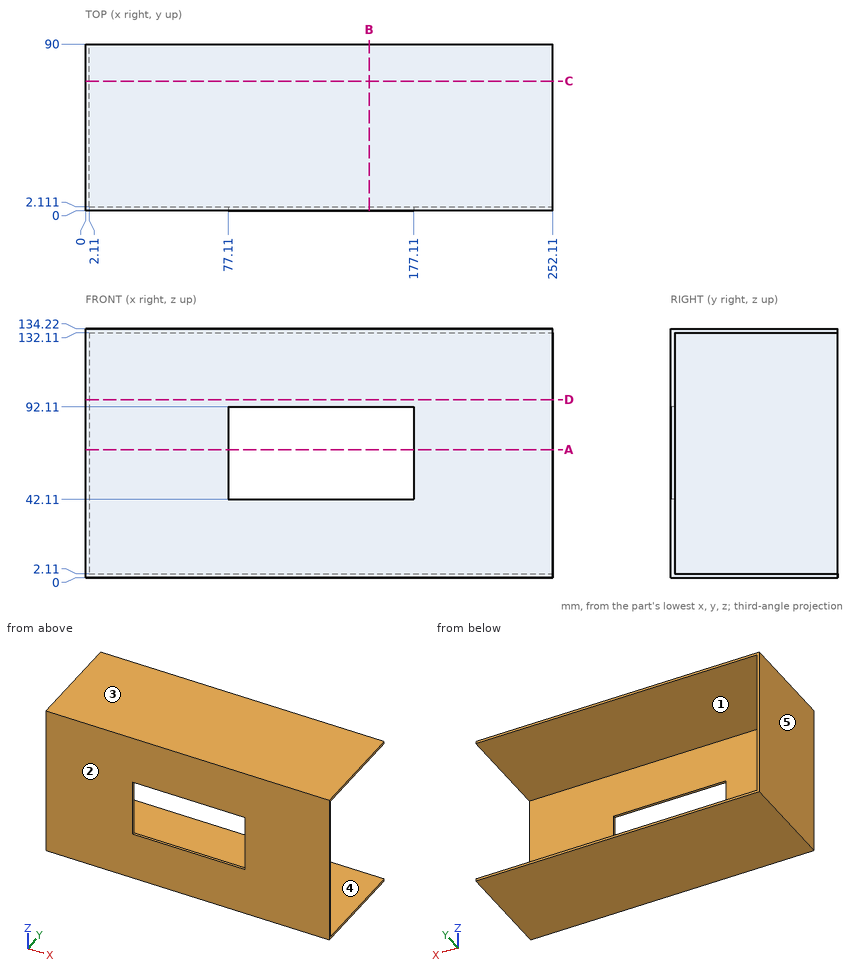
Job drawing, mm, ordinate dimensions from the low corner. One solid piece. A direction names the side the tool comes from. Give positions to 0.01 mm unless a question says otherwise; leave off trailing zeros. Loops run counter-clockwise (first coordinate to the right, second up) from the corner with the lowest first, then second, coordinate; pieces in that order, holes last. Notation, with made-up numbers: M 28,42.5 L 83,42.5 A21 cw 83,60.5 Z; hole C 56.25,-7.75 d6. An arc over 180 degrees is marked long. Answer in a Markdown table with one row per item. Add a question column.
Item 1: Band-saw the part on B-B on x = 153. Give the cut face in (y, z), then the cut area to 3 significant figures.
Item 2: Drop a flat-ended pin along its axis: P1, Ø8, axis at x = 134, z = 37, coming from the +Y side. Give the stop position or say it passes through.
Item 3: Band-saw the part on A-A on z = 69. Give the cut face in (x, y).
Item 4: Band-saw the part on D-D on z = 96. Give the cut face in (x, y), then the cut area to 3 significant figures.
Item 5: Tool access for the marked faces 1 and 2: list every direction of +Z, -Z, +X, -X, +Y, -Y with a clear straight run to the whole face (end or side of a thin tool).
Item 6: Band-saw the part on C-C on y = 70. Give the cut face in (x, z).
Item 7: Probe probe 1 along Z at (x, y) = (230, 31.5); probe 2 along Y at (x, z) = (217.5, 84.5). List the from-to ranges inside material, lowest first.
Item 8: Mould opens along Z. For the marked faces 3, 4 and 5 say: +Z half, -Z half, draft (parallel to the pull), parting line (faces both ways), or undercut.
Reply:
| question | item | result |
|---|---|---|
| 1 | outline | M 0,0 L 90,0 L 90,2.11 L 2.11,2.11 L 2.11,42.11 L 0,42.11 Z; M 0,92.11 L 2.11,92.11 L 2.11,132.11 L 90,132.11 L 90,134.22 L 0,134.22 Z |
| 1 | area | 549 mm^2 |
| 2 | P1 | stops at y = 2.11 |
| 3 | outline | M 0,0 L 77.11,0 L 77.11,2.11 L 2.11,2.11 L 2.11,90 L 0,90 Z; M 177.11,0 L 252.11,0 L 252.11,2.11 L 177.11,2.11 Z |
| 4 | outline | M 0,0 L 252.11,0 L 252.11,2.11 L 2.11,2.11 L 2.11,90 L 0,90 Z |
| 4 | area | 718 mm^2 |
| 5 | face 1 | +X, +Y |
| 5 | face 2 | +Z, -Z, +X, -X, -Y |
| 6 | outline | M 0,0 L 252.11,0 L 252.11,2.11 L 2.11,2.11 L 2.11,132.11 L 252.11,132.11 L 252.11,134.22 L 0,134.22 Z |
| 7 | probe 1 | z = 0 to 2.11, 132.11 to 134.22 |
| 7 | probe 2 | y = 0 to 2.11 |
| 8 | face 3 | +Z half |
| 8 | face 4 | undercut |
| 8 | face 5 | draft |
